Autodesk Inventor part; units mm, degrees
ref_plane "YZ Plane" through (0, 0, 0) normal (1, 0, 0) x (0, 1, 0)
ref_plane "XZ Plane" through (0, 0, 0) normal (0, 1, 0) x (-1, 0, 0)
ref_plane "XY Plane" through (0, 0, 0) normal (0, 0, 1) x (1, 0, 0)
sketch "Sketch1" plane through (0, 0, 0) normal (0, 1, 0) x (-1, 0, 0)
  line L0 (-30.1299, 69.45) -> (30.245, 69.45)
  line L1 (30.245, -69.45) -> (-30.1299, -69.45)
  circle A0 centre (0, 0) radius 37.5
  arc A1 (-30.1299, 69.45) -> (-30.1299, -69.45) centre (0, 0) ccw
  arc A2 (30.245, -69.45) -> (30.245, 69.45) centre (0, 0) ccw
  circle A3 centre (0, -58.5) radius 6
  circle A4 centre (0, -58.5) radius 3.25
  circle A5 centre (0, 0) radius 45.75 construction
  circle A6 centre (50.6625, 29.25) radius 6
  circle A7 centre (50.6625, 29.25) radius 3.25
  circle A8 centre (-50.6625, 29.25) radius 6
  circle A9 centre (-50.6625, 29.25) radius 3.25
  line L2 (87.5, -76) -> (-87.5, -76)
  line L3 (-87.5, -76) -> (-87.5, 76)
  line L4 (-87.5, 76) -> (87.5, 76)
  line L5 (87.5, 76) -> (87.5, -76)
  point P0 (-87.5, 0)
  point P1 (0, -76)
  dimension "d1" = 75
  dimension "d2" = 69.45
  dimension "d3" = 58.5
  dimension "d4" = 12
  dimension "d5" = 6.5
  dimension "d8" = 360
  dimension "d57" = 75.75
  dimension "d58" = 69.45
  dimension "d59" = 69.45
  dimension "d69" = 152
  dimension "d70" = 175
extrude "Extrusion1" add sketch "Sketch1" along normal blind 5 contours L0 A2 L1 A1 | A3 | A6 | A8 | L2 L3 L4 L5
sketch "Sketch2" plane through (0, 5, 0) normal (0, 1, 0) x (1, 0, 0)
  circle A0 centre (0, 58.5) radius 3.25
  circle A1 centre (0, 58.5) radius 6
  circle A2 centre (50.6625, -29.25) radius 3.25
  circle A3 centre (50.6625, -29.25) radius 6
  circle A4 centre (-50.6625, -29.25) radius 3.25
  circle A5 centre (-50.6625, -29.25) radius 6
  point P0 (0, 0)
  dimension "d12" = 12
  dimension "d13" = 12
  dimension "d14" = 12
extrude "Extrusion2" cut sketch "Sketch2" against normal blind 6.5
sketch "Sketch11" plane through (0, 5, 0) normal (0, 1, 0) x (1, 0, 0)
  circle A0 centre (-50.6625, -29.25) radius 6
  circle A1 centre (0, 58.5) radius 6
  circle A2 centre (50.6625, -29.25) radius 6
  circle A3 centre (0, 0) radius 37.5
  line L0 (87.5, 76) -> (-87.5, 76)
  line L1 (-87.5, 76) -> (-87.5, -76)
  line L2 (-87.5, -76) -> (87.5, -76)
  line L3 (87.5, -76) -> (87.5, 76)
  line L4 (-87.5, 76) -> (-67.5, 76)
  line L5 (-67.5, 76) -> (-67.5, -76)
  line L6 (-67.5, -76) -> (-87.5, -76)
  line L7 (-87.5, -76) -> (-87.5, 76)
  line L8 (87.5, 76) -> (-87.5, 76)
  line L9 (87.5, -76) -> (-87.5, -76)
  line L10 (87.5, 76) -> (67.5, 76)
  line L11 (67.5, 76) -> (67.5, -76)
  line L12 (67.5, -76) -> (87.5, -76)
  line L13 (87.5, -76) -> (87.5, 76)
  point P0 (0, 0)
  dimension "d71" = 20
  dimension "d72" = 20
extrude "Extrusion11" add sketch "Sketch11" along normal blind 10 contours L3 L2 L11 L0 | L5 L2 L1 L0
fillet "Fillet9" radius 5 4 edges at (-67.5, 15, 0) (-87.5, 15, 0) (67.5, 15, 0) (87.5, 15, 0)
equation "\"d2\" = d59"
properties part number "soporte inferior ridgid -2"
Geometry check sheet. Reference: the model listing, model coordinates, mm. A direction names the side the tool comes from. Give positions to 0.01 mm unless a question says otherwise; leave off trailing zeros. Order: outer loops, then holes, each group sorted by start corner. A loop starts at its lowest first (then second) coordinate and runs counter-clockwise, first axis right, second up. Notation, with made-up numbers: (-4.75, -1.75) - (1.25, -1.75) arc R21 ccw to (1.25, 23.25) - close; hole circle Ø1 at (52.5, -39). An arc over 180 degrees is marked (long way). Write item = value, one per line. Start each with the question number.
1) Draft check along Z on faces 1 (the flat face through (-1, 4, -76)), 2 (the flat face through (21, 0, 35)), 3 (the cylindrical face through (45.9, 2.5, 32.9)). Enter one of: released by +Z, released by -Z, zero draft, split by the parting line, or undercut.
2) Gauge pin test, flat ends, axial feed: pin 1 Ø9.5 at (x, z) = (0, -58.5) entering from +Y; pin 2 Ø2 at (y, z) = (13.5, 1) entering from +X; pin 3 Ø8 at (x, z) = (-2.5, -35) entering from +Y. Record the tip position at first contact, or that the pin passes through.
3) Section check B-B (z = -58.5). Enter the section's corners in (x, y), then the cut area to 3 significant figures.
4) Scan lines: L1, parallel to Z at x = 0, y = 2.85; L2, parallel to X at y = 2.2, z = -58.5; L3, parallel to X at y = 3.55, z = 29.25. Record each from-to range of solid material in increasing order.
5) Section check C-C (x = 0). Enter the section's corners in (y, z).
6) Access from +Z, -Z, +X, -X, +Y, -Y to the whole of each face (thin tool, end or side, straight path). Record for faces 4 (the flat face through (-87.5, 5, 1)), 5 (the flat face through (-14, 5, 35)).
7) Section check D-D (x = 54). Enter the section's corners in (y, z).
8) Section check A-A (y = 7.75). Enter the section's corners in (x, z).
Geometry check:
q1.face_1 = released by -Z
q1.face_2 = zero draft
q1.face_3 = undercut
q2.pin_1 = through
q2.pin_2 = 86.83
q2.pin_3 = 5
q3.outline = (-87.5, 0) - (-6, 0) - (-6, 5) - (-67.5, 5) - (-67.5, 10) arc R5 ccw to (-72.5, 15) - (-82.5, 15) arc R5 ccw to (-87.5, 10) - close; (6, 0) - (87.5, 0) - (87.5, 10) arc R5 ccw to (82.5, 15) - (72.5, 15) arc R5 ccw to (67.5, 10) - (67.5, 5) - (6, 5) - close
q3.area = 1,190 mm2
q4.L1 = -76 to -64.5, -52.5 to -37.5, 37.5 to 76
q4.L2 = -87.5 to -6, 6 to 87.5
q4.L3 = -87.5 to -56.66, -44.66 to -23.47, 23.47 to 44.66, 56.66 to 87.5
q5.outline = (0, -76) - (5, -76) - (5, -64.5) - (0, -64.5) - close; (0, -52.5) - (5, -52.5) - (5, -37.5) - (0, -37.5) - close; (0, 37.5) - (5, 37.5) - (5, 76) - (0, 76) - close
q6.face_4 = +Z, -Z, -X, +Y, -Y
q6.face_5 = +Z, -Z, +Y
q7.outline = (0, -76) - (5, -76) - (5, 24.26) - (0, 24.26) - close; (0, 34.24) - (5, 34.24) - (5, 76) - (0, 76) - close
q8.outline = (-87.5, -76) - (-67.5, -76) - (-67.5, 76) - (-87.5, 76) - close; (67.5, -76) - (87.5, -76) - (87.5, 76) - (67.5, 76) - close
